CAD build for the part. Positions are in the model's coordinates, mm. Coordinates: 2 decimals unless noted, no trailing zeros. Loops run counter-clockwise (first coordinate to the right, second up) from the corner with the lowest first, then second, coordinate; pieces in that order, holes last. Notation, with made-up numbers: (-27.75, -37) -> (21.25, -37) arc R34 cw to (21.25, -5) -> close; hole circle Ø4 at (28, 25). An arc over 180 degrees is marked (long way). Return JSON: item names as keys, results as strings. Group by question number.
(1) Saw through at B-B on y = 177.8. Write the cut outline in (x, z) (3 decimals), then the cut area to 3 significant figures.
(2) Saw through at C-C on y = 0. Write the cut outline in (x, z) (3 decimals).
(3) Probe L1, parallel to Y at x = -177.8, z = 0 (3 decimals); L2, parallel to X at y = -176.5, z = 0.5. List the from-to ranges inside material, lowest first.
(4) Saw through at A-A on x = 0. Write the cut outline in (y, z) (3 decimals).
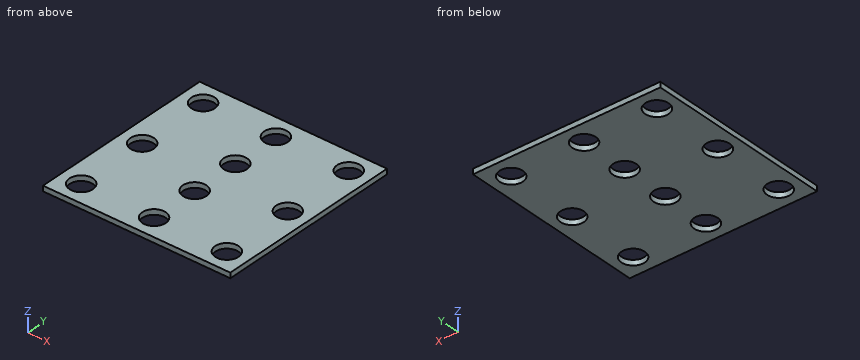
```python
from build123d import *

# Parameters (mm, degrees)
F0_W     = 457.2
F0_H     = 457.2
F2_DEPTH = 6.35
F1_R     = 28.575
F3_DEPTH = 12.7


with BuildPart() as f2:
    # F0 (on Top) → F2 (new body, symmetric)
    with BuildSketch(Plane.XY):
        Rectangle(F0_W, F0_H)
    extrude(amount=F2_DEPTH, both=True)

    # F1 (on face) → F3 (cut, symmetric)
    with BuildSketch(Plane.XY):
        with Locations((-177.8, 177.8)):
            Circle(F1_R)
        with Locations((0, 177.8)):
            Circle(F1_R)
        with Locations((177.8, 177.8)):
            Circle(F1_R)
        with Locations((177.8, 0)):
            Circle(F1_R)
        with Locations((177.8, -177.8)):
            Circle(F1_R)
        with Locations((-177.8, 0)):
            Circle(F1_R)
        with Locations((-177.8, -177.8)):
            Circle(F1_R)
        with Locations((0, 59.266667)):
            Circle(F1_R)
        with Locations((0, -59.266667)):
            Circle(F1_R)
        with Locations((0, -177.8)):
            Circle(F1_R)
    extrude(amount=F3_DEPTH, both=True, mode=Mode.SUBTRACT)


solid = f2.part
```
Geometry results:
{
 "1": {"outline": "(-228.6, -6.35) -> (-206.375, -6.35) -> (-206.375, 6.35) -> (-228.6, 6.35) -> close; (-149.225, -6.35) -> (-28.575, -6.35) -> (-28.575, 6.35) -> (-149.225, 6.35) -> close; (28.575, -6.35) -> (149.225, -6.35) -> (149.225, 6.35) -> (28.575, 6.35) -> close; (206.375, -6.35) -> (228.6, -6.35) -> (228.6, 6.35) -> (206.375, 6.35) -> close", "area": "3,630 mm²"},
 "2": {"outline": "(-228.6, -6.35) -> (-206.375, -6.35) -> (-206.375, 6.35) -> (-228.6, 6.35) -> close; (-149.225, -6.35) -> (149.225, -6.35) -> (149.225, 6.35) -> (-149.225, 6.35) -> close; (206.375, -6.35) -> (228.6, -6.35) -> (228.6, 6.35) -> (206.375, 6.35) -> close"},
 "3": {"L1": "-228.6 to -206.375, -149.225 to -28.575, 28.575 to 149.225, 206.375 to 228.6", "L2": "-228.6 to -206.35, -149.25 to -28.55, 28.55 to 149.25, 206.35 to 228.6"},
 "4": {"outline": "(-228.6, -6.35) -> (-206.375, -6.35) -> (-206.375, 6.35) -> (-228.6, 6.35) -> close; (-149.225, -6.35) -> (-87.842, -6.35) -> (-87.842, 6.35) -> (-149.225, 6.35) -> close; (-30.692, -6.35) -> (30.692, -6.35) -> (30.692, 6.35) -> (-30.692, 6.35) -> close; (87.842, -6.35) -> (149.225, -6.35) -> (149.225, 6.35) -> (87.842, 6.35) -> close; (206.375, -6.35) -> (228.6, -6.35) -> (228.6, 6.35) -> (206.375, 6.35) -> close"}
}
